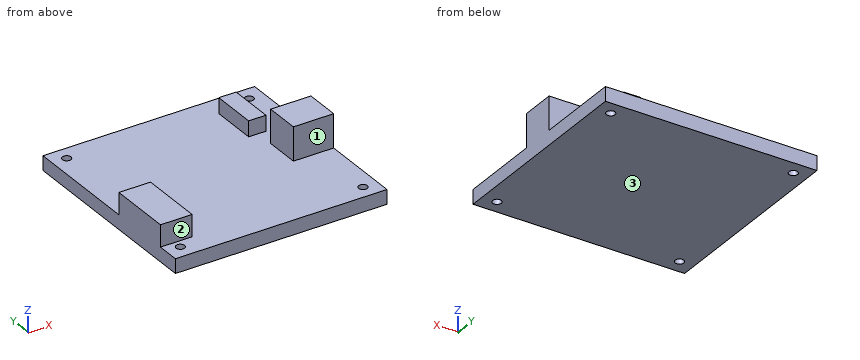
from build123d import *

# Parameters (mm, degrees)
SKETCH1_W           = 73.6
SKETCH1_H           = 71
BOSS_EXTRUDE1_DEPTH = 5
SKETCH2_R           = 1.5
CUT_EXTRUDE1_DEPTH  = 6
SKETCH3_W           = 11
SKETCH3_H           = 22.3
BOSS_EXTRUDE2_DEPTH = 7.54
SKETCH4_W           = 14
SKETCH4_H           = 12.2
BOSS_EXTRUDE3_DEPTH = 11.6
SKETCH5_W           = 6
SKETCH5_H           = 16
BOSS_EXTRUDE4_DEPTH = 5.4


with BuildPart() as part:
    # Sketch1 → Boss-Extrude1 (new body)
    with BuildSketch(Plane.XY):
        with Locations((36.8, 35.5)):
            Rectangle(SKETCH1_W, SKETCH1_H)
    extrude(amount=BOSS_EXTRUDE1_DEPTH)

    # Sketch2 → Cut-Extrude1 (cut, through all)
    with BuildSketch(Plane.XY.offset(5)):
        with Locations((5, 5)):
            Circle(SKETCH2_R)
        with Locations((68.5, 5)):
            Circle(SKETCH2_R)
        with Locations((68.5, 66)):
            Circle(SKETCH2_R)
        with Locations((5, 66)):
            Circle(SKETCH2_R)
    extrude(amount=-CUT_EXTRUDE1_DEPTH, mode=Mode.SUBTRACT)

    # Sketch3 → Boss-Extrude2 (add)
    with BuildSketch(Plane.XY.offset(5)):
        with Locations((5.5, 19.15)):
            Rectangle(SKETCH3_W, SKETCH3_H)
    extrude(amount=BOSS_EXTRUDE2_DEPTH)

    # Sketch4 → Boss-Extrude3 (add)
    with BuildSketch(Plane.XY.offset(5)):
        with Locations((66.6, 34.7)):
            Rectangle(SKETCH4_W, SKETCH4_H)
    extrude(amount=BOSS_EXTRUDE3_DEPTH)

    # Sketch5 → Boss-Extrude4 (add)
    with BuildSketch(Plane.XY.offset(5)):
        with Locations((59.3, 55.5)):
            Rectangle(SKETCH5_W, SKETCH5_H)
    extrude(amount=BOSS_EXTRUDE4_DEPTH)


solid = part.part
Geometry check sheet. Reference: the model listing, model coordinates, mm. Face numbers are marked on the shaded views. A direction names the side the tool comes from. Give positions to 0.01 mm unless a question says otherwise; leave off trailing zeros. Write each loop counter-clockwise with the first axis right and the second up, starting at its lowest first coordinate (ties: lowest second). Pieces come first, ordered by that corner, then holes. Notation, with made-up numbers: M 73,-38 L 88,-38 A11 cw 88,-20 Z; hole C 72.25,21.25 d2. An arc over 180 degrees is marked long. Answer as CSV lines item,"result". Start each with the question number.
Q1. Go/stop test with flat-tipped pins: pin 1 (4 mm diameter, centred on x = 5, y = 66, fed in from +Z); pin 2 (2.5 mm diameter, centred on x = 68.5, y = 66, fed in from +Z) (3 decimals); pin 3 (12 mm diameter, centred on x = 3, y = 19.5, fed in from +Z); pin 4 (9.5 mm diameter, centred on x = 65.5, z = 11, fed in from +Y). Record where each tip stops, or that it passes through.
Q2. Material ranges on L1, parallel to X at y = 66, z = 1.15; L2, parallel to Y at x = 68.5, z = 1.2; L3, parallel to X at y = 29.5, z = 12, recorded low to high.
Q3. Section check D-D, the plane y = 38.5. Record the cut outline in (x, z).
Q4. Section check A-A, the plane y = 66. Record the cut outline in (x, z).
Q5. Section check B-B, the plane x = 68.5. Record the cut outline in (y, z), then the cut area to 3 significant figures.
Q6. Tool access check on the marked faces 1, 2 and 3. Record the directions out of +Z, -Z, +X, -X, +Y, -Y that give a thin tool (end or side, any length) a straight path to the whole face; none if there is none.
Q7. Section check C-C, the plane x = 61. Record the cut outline in (y, z).
Geometry says:
1,pin 1,"z = 5"
1,pin 2,"through"
1,pin 3,"z = 12.54"
1,pin 4,"y = 63.5"
2,L1,"0 to 3.5, 6.5 to 67, 70 to 73.6"
2,L2,"0 to 3.5, 6.5 to 64.5, 67.5 to 71"
2,L3,"0 to 11, 59.6 to 73.6"
3,outline,"M 0,0 L 73.6,0 L 73.6,16.6 L 59.6,16.6 L 59.6,5 L 0,5 Z"
4,outline,"M 0,0 L 3.5,0 L 3.5,5 L 0,5 Z; M 6.5,0 L 67,0 L 67,5 L 6.5,5 Z; M 70,0 L 73.6,0 L 73.6,5 L 70,5 Z"
5,outline,"M 0,0 L 3.5,0 L 3.5,5 L 0,5 Z; M 6.5,0 L 64.5,0 L 64.5,5 L 40.8,5 L 40.8,16.6 L 28.6,16.6 L 28.6,5 L 6.5,5 Z; M 67.5,0 L 71,0 L 71,5 L 67.5,5 Z"
5,area,"467 mm^2"
6,face 1,"+Z, +X, -Y"
6,face 2,"+Z, +X, -X, -Y"
6,face 3,"-Z, +X, -X, +Y, -Y"
7,outline,"M 0,0 L 71,0 L 71,5 L 63.5,5 L 63.5,10.4 L 47.5,10.4 L 47.5,5 L 40.8,5 L 40.8,16.6 L 28.6,16.6 L 28.6,5 L 0,5 Z"
